Geometry: final body of the model. Coordinates: model frame, mm. A direction names the side the tool comes from. Give positions to 0.01 mm unless a question says otherwise; leave off trailing zeros. Order: outer loops, then holes, each group sorted by start corner. A loop starts at its lowest first (then second) coordinate and runs counter-clockwise, first axis right, second up. Notation, with made-up numbers: (72, -7.75) -> (125, -7.75) arc R19 cw to (125, 12.25) -> close; hole circle Ø1 at (48, -24). An arc over 180 degrees is marked (long way). Answer in a Markdown table with one row per item. Add a question column.
Q1. Cut plane A-A on z = -3. Return the cut outline in (x, y), and give its area (3 significant figures).
Q2. Pull-direction query (X, two-part tool) for faces 4 (the face through (-2.57, 1.48, -24.56)), 5 (the face through (15.14, 1.52, -24.44)), 6 (the face through (-4, 1, -5)), 7 (the face through (55, 2, -2)); classes: +X half, -X half, draft (parallel to the pull), parting line (faces both ways), or undercut.
Q3. Contact query for flat-ended pins moving along their axis: P1, Ø8, axis at x = 67.5, z = -3.5, coming from the -Y side; P2, Ø1, axis at y = 2, z = -23, coming from the +X side; P3, Ø0.9, axis at x = -6, y = 2, coming from the -Z side; P4, Ø0.9, axis at x = 36.5, y = 1.5, coming from the +Z side. Output: stop coordinate, or through.
Q4. Set-up query: faces 1 (the face through (72, 1, -5)), 2 (the face through (20, 1, -2)), 3 (the face through (-7, 1, -25)). Return all of +Z, -Z, +X, -X, +Y, -Y with unobstructed straight access to the full face (end or side cutting, diameter ignored); none if empty.
Q5. Cut plane B-B on y = 0.6. Return the cut outline in (x, z), and give its area (3 significant figures).
Q6. Cut plane C-C on x = 38. Return the cut outline in (y, z), and give its area (3 significant figures).
Q7. Cut plane D-D on z = -12. Return the cut outline in (x, y), and give its area (3 significant figures).
Q8. Line query: line 1 along X through (y, z) = (1.1, -2); line 2 along X through (y, z) = (2.05, -25.5); line 3 along Z through (x, y) = (67.5, 2.2). Output: solid intervals per line, ascending. Write a range as from..to.
from build123d import *

# Parameters (mm, degrees)
BOSS_EXTRUDE1_DEPTH = 3
SKETCH2_W           = 10
SKETCH2_H           = 5
BOSS_EXTRUDE2_DEPTH = 3
BOSS_EXTRUDE3_DEPTH = 3


with BuildPart() as part:
    # Sketch1 → Boss-Extrude1 (new body)
    with BuildSketch(Plane(origin=(0, 0, 0), x_dir=(1, 0, 0), z_dir=(0, 1, 0))):
        Polygon((20, 0), (20, 5), (80, 5), (80, 10), (-5.069227294, 25), (-8.069227294, 25), (-8.069227294, 5), (0, 5), (0, 0), align=None)
    extrude(amount=BOSS_EXTRUDE1_DEPTH)

    # Sketch2 → Boss-Extrude2 (add)
    with BuildSketch(Plane(origin=(0, 3, 0), x_dir=(1, 0, 0), z_dir=(0, 1, 0))):
        with Locations((60, 2.5)):
            Rectangle(SKETCH2_W, SKETCH2_H)
    extrude(amount=-BOSS_EXTRUDE2_DEPTH)

    # Sketch3 → Boss-Extrude3 (add)
    with BuildSketch(Plane(origin=(0, 3, 0), x_dir=(1, 0, 0), z_dir=(0, 1, 0))):
        Polygon((-0.145188529, 24.131759112), (14.626927766, 21.527036447), (15.668816832, 27.435882965), (0.896700537, 30.04060563), align=None)
    extrude(amount=-BOSS_EXTRUDE3_DEPTH)


solid = part.part
Completed:
| question | item | result |
|---|---|---|
| 1 | outline | (0, 0) -> (20, 0) -> (20, 3) -> (0, 3) -> close; (55, 0) -> (65, 0) -> (65, 3) -> (55, 3) -> close |
| 1 | area | 90.0 mm² |
| 2 | face 4 | undercut |
| 2 | face 5 | +X half |
| 2 | face 6 | draft |
| 2 | face 7 | undercut |
| 3 | P1 | stops at y = 0 |
| 3 | P2 | stops at x = 14.97 |
| 3 | P3 | stops at z = -25 |
| 3 | P4 | stops at z = -5 |
| 4 | face 1 | +Z, +X, +Y, -Y |
| 4 | face 2 | +Z, +Y, -Y |
| 4 | face 3 | -Z, -X, +Y, -Y |
| 5 | outline | (-8.07, -25) -> (-5.07, -25) -> (-0.15, -24.13) -> (0.9, -30.04) -> (15.67, -27.44) -> (14.63, -21.53) -> (80, -10) -> (80, -5) -> (65, -5) -> (65, 0) -> (55, 0) -> (55, -5) -> (20, -5) -> (20, 0) -> (0, 0) -> (0, -5) -> (-8.07, -5) -> close |
| 5 | area | 1,360 mm² |
| 6 | outline | (0, -17.41) -> (3, -17.41) -> (3, -5) -> (0, -5) -> close |
| 6 | area | 37.2 mm² |
| 7 | outline | (-8.07, 0) -> (68.66, 0) -> (68.66, 3) -> (-8.07, 3) -> close |
| 7 | area | 230 mm² |
| 8 | line 1 | x = 0..20, 55..65 |
| 8 | line 2 | x = 0.1..15.33 |
| 8 | line 3 | z = -12.2..-5 |
